Job drawing, mm, ordinate dimensions from the low corner. One solid piece. Round coordinates to 2 decimals unless told otherwise and drop trailing zeros. Loops run counter-clockwise (first coordinate to the right, second up) from the corner with the lowest first, then second, coordinate; pieces in that order, holes last. Notation, with made-up numbers: M -38,73.5 L -30,73.5 A28 ccw -30,107.5 Z; hole C 32.25,89 d5. An arc over 180 degrees is marked long. Put each result on its own line as item: value. Start each with the question number.
1) Slice it at A-A on x = 5.08. Give the cut face in (y, z).
2) Probe line 1 along X through (y, z) = (84, 40.5) (1 decimal); line 2 along X through (y, z) = (80, 22) (1 decimal); line 3 along X through (y, z) = (89.5, 67.5). List the from-to ranges inside material, lowest first.
3) Slice it at B-B on z = 59.5. Give the cut face in (x, y).
4) Drop flat-ended pins along their axis: pin 1 Ø6 at (x, z) = (13.5, 41) entering from -Y; pin 2 Ø14 at (y, z) = (91, 42) entering from -X; pin 3 Ø2.5 at (x, z) = (15, 55.5) entering from +Y. Give the stop position or say it passes through.
5) Slice it at D-D on x = 161. Give the cut face in (y, z), then the cut area to 4 significant figures.
6) Slice it at C-C on y = 50.8. Give the cut face in (x, z).
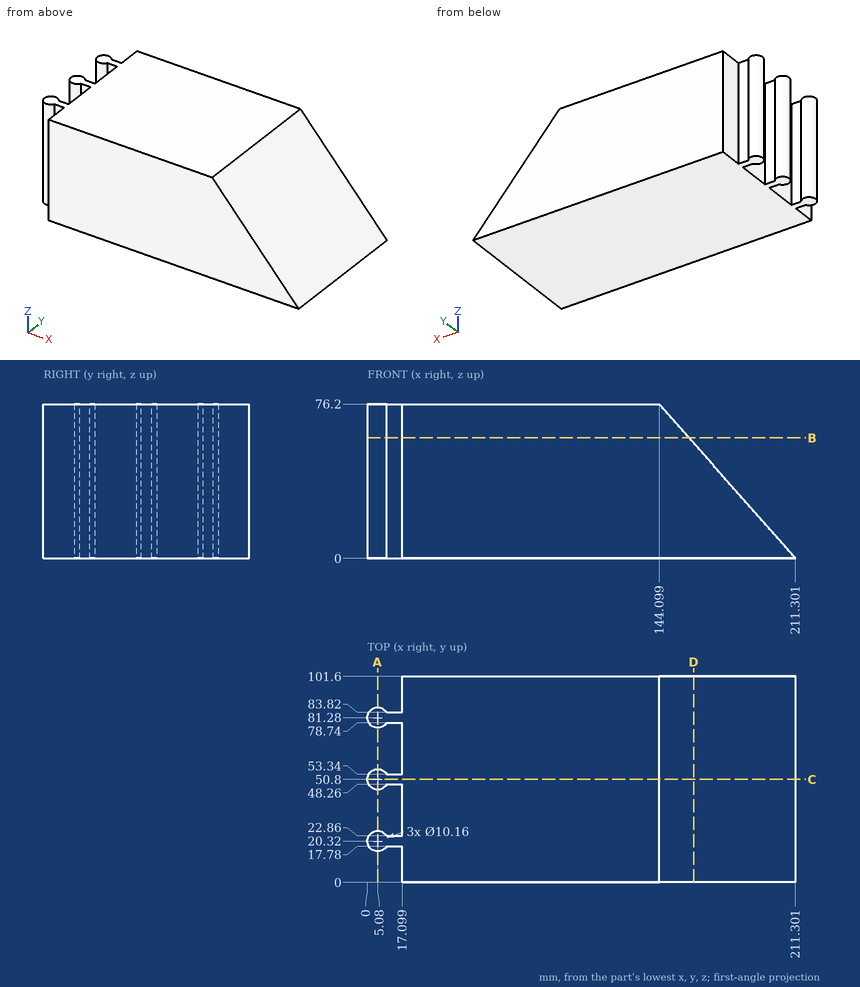
Recorded:
1. outline: M 15.24,0 L 25.4,0 L 25.4,76.2 L 15.24,76.2 Z; M 45.72,0 L 55.88,0 L 55.88,76.2 L 45.72,76.2 Z; M 76.2,0 L 86.36,0 L 86.36,76.2 L 76.2,76.2 Z
2. line 1: x = 0.8 to 9.4, 17.1 to 175.6
2. line 2: x = 0.2 to 191.9
2. line 3: x = 17.1 to 151.77
3. outline: M 9.48,17.78 L 17.1,17.78 L 17.1,0 L 158.83,0 L 158.83,101.6 L 17.1,101.6 L 17.1,83.82 L 9.48,83.82 A5.08 ccw long 9.48,78.74 L 17.1,78.74 L 17.1,53.34 L 9.48,53.34 A5.08 ccw long 9.48,48.26 L 17.1,48.26 L 17.1,22.86 L 9.48,22.86 A5.08 ccw long Z
4. pin 1: stops at y = 17.78
4. pin 2: stops at x = 0.79
4. pin 3: stops at y = 83.82
5. outline: M 0,0 L 101.6,0 L 101.6,57.04 L 0,57.04 Z
5. area: 5,795 mm2
6. outline: M 0,0 L 211.3,0 L 144.1,76.2 L 0,76.2 Z
